Source: CAD feature listing. Evaluate the final solid. Frame: model axes, mm. Face numbers are marked on the shaded views. A direction names the side the tool comes from. Coordinates: 2 decimals unless noted, no trailing zeros. Order: outer loops, then holes, each group sorted by start corner. A loop starts at its lowest first (then second) coordinate and runs counter-clockwise, first axis right, second up.
```python
from build123d import *

# Parameters (mm, degrees)
SKETCH2_W           = 40
SKETCH2_H           = 6
SKETCH2_R           = 2
BOSS_EXTRUDE1_DEPTH = 3
SKETCH3_W           = 22
SKETCH3_H           = 6
BOSS_EXTRUDE2_DEPTH = 22
CUT_EXTRUDE1_REACH  = 49.55
SKETCH4_R           = 9.75


with BuildPart() as part:
    # Sketch2 → Boss-Extrude1 (new body)
    with BuildSketch(Plane(origin=(0, 0, 0), x_dir=(1, 0, 0), z_dir=(0, 1, 0))):
        with Locations((-20, 3)):
            Rectangle(SKETCH2_W, SKETCH2_H)
        with Locations(Location((-3, 3, 0), (0, 0, 270))):
            Circle(SKETCH2_R, mode=Mode.SUBTRACT)
    extrude(amount=BOSS_EXTRUDE1_DEPTH)

    # Sketch3 → Boss-Extrude2 (add)
    with BuildSketch(Plane(origin=(0, 3, 0), x_dir=(1, 0, 0), z_dir=(0, 1, 0))):
        with Locations((-29, 3)):
            Rectangle(SKETCH3_W, SKETCH3_H)
    extrude(amount=BOSS_EXTRUDE2_DEPTH)

    # Sketch4 → Cut-Extrude1 (cut, up to next)
    with BuildSketch(Plane(origin=(0, 0, -6), x_dir=(-1, 0, 0), z_dir=(0, 0, -1)), mode=Mode.PRIVATE) as cut_extrude1_sk1:
        with Locations((29, 14)):
            Circle(SKETCH4_R)
    cut_extrude1_tool1 = extrude(cut_extrude1_sk1.sketch, amount=-CUT_EXTRUDE1_REACH, mode=Mode.PRIVATE) & part.part
    add(cut_extrude1_tool1.solids().sort_by_distance((-29, 14, -6))[0], mode=Mode.SUBTRACT)


solid = part.part
```
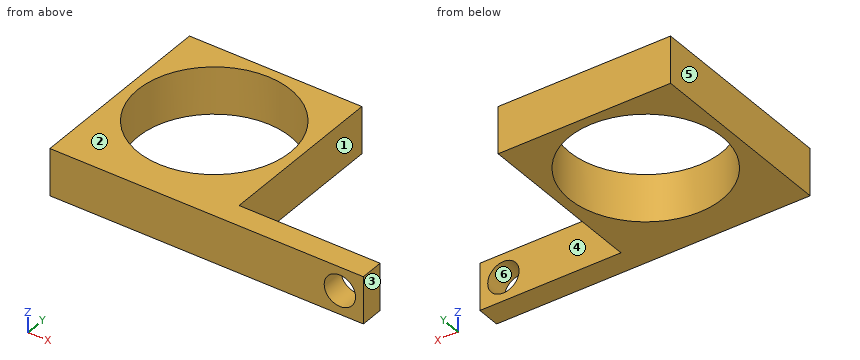
1. Draft query along X for the marked faces 3, 4, 5 and 6. Return one class per face: released by +X, released by -X, zero draft, split by the parting line, or undercut.
Findings:
face 3: released by +X
face 4: zero draft
face 5: released by -X
face 6: undercut
2. Section query D-D on y = 1.5. Return loops of the section in (x, z), plus the area to 3 significant figures.
Findings:
outline: (-40, -6) - (0, -6) - (0, 0) - (-40, 0) - close; hole circle Ø4 at (-3, -3)
area: 227 mm2
3. Access query for the marked faces 1 and 2. Directions: +Z, -Z, +X, -X, +Y, -Y. A direction counts if a zero-diameter tool reaches every point of the face in a straight line with its end or side. Return the directions, or none.
Findings:
face 1: +Z, -Z, +X, +Y
face 2: +Z, +X, -X, +Y, -Y
4. Ray query, line 1 (X direction, y = 0.8, z = -3); line 2 (Y direction, x = -29, z = -1.2); line 3 (Y direction, x = -14.5, z = -3.9). Return the intervals inside material, ascending.
Findings:
line 1: x = -40 to -5, -1 to 0
line 2: y = 0 to 4.25, 23.75 to 25
line 3: y = 0 to 3
5. Pin query (flat end, axial travel): P1, Ø1.5, axis at y = 11, z = -4.5, coming from the +X side. Return the tip coordinate at first contact, or that it passes through.
Findings:
P1: stops at x = -18
6. Section query C-C on x = -3. Return loops of the section in (y, z).
Findings:
outline: (0, -6) - (3, -6) - (3, -5) - (0, -5) - close; (0, -1) - (3, -1) - (3, 0) - (0, 0) - close
7. Section query B-B on z = -3. Return loops of the section in (x, y), plus the area to 3 significant figures.
Findings:
outline: (-40, 0) - (-5, 0) - (-5, 3) - (-18, 3) - (-18, 25) - (-40, 25) - close; (-1, 0) - (0, 0) - (0, 3) - (-1, 3) - close; hole circle Ø19.5 at (-29, 14)
area: 293 mm2
8. Section query A-A on y = 14. Return loops of the section in (x, z).
Findings:
outline: (-40, -6) - (-38.75, -6) - (-38.75, 0) - (-40, 0) - close; (-19.25, -6) - (-18, -6) - (-18, 0) - (-19.25, 0) - close
